Geometry check sheet. Reference: the model listing, model coordinates, mm. A direction names the side the tool comes from. Round coordinates to 2 decimals unless told otherwise and drop trailing zeros. Order: outer loops, then holes, each group sorted by start corner. A loop starts at its lowest first (then second) coordinate and runs counter-clockwise, first axis right, second up.
```python
from build123d import *

# Parameters (mm, degrees)
SKETCH_1_W          = 108
SKETCH_1_H          = 70
SKETCH_1_W_2        = 102
SKETCH_1_H_2        = 64
EXTRUDE_1_DEPTH     = 5
EXTRUDE_8_DEPTH     = 3
SKETCH_4_W          = 20
SKETCH_4_H          = 18
EXTRUDE_9_DEPTH     = 20
SKETCH_5_R          = 6.2
CUT_EXTRUDE_1_DEPTH = 76.7627877
FILLET_2_R          = 1
EXTRUDE_10_DEPTH    = 1
EXTRUDE_11_DEPTH    = 3
FILLET_3_R          = 3
SKETCH_8_R          = 10
CUT_EXTRUDE_2_DEPTH = 5
SKETCH_9_R          = 1
EXTRUDE_12_DEPTH    = 4
FILLET_4_R          = 3
FILLET_5_R          = 1
EXTRUDE_13_DEPTH    = 3
SKETCH_12_R         = 1
EXTRUDE_15_DEPTH    = 3


with BuildPart() as part:
    # 草图1 → 凸台-拉伸1 (new body)
    with BuildSketch(Plane(origin=(0, 0, 0), x_dir=(1, 0, 0), z_dir=(0, 1, 0))):
        Rectangle(SKETCH_1_W, SKETCH_1_H)
        Rectangle(SKETCH_1_W_2, SKETCH_1_H_2, mode=Mode.SUBTRACT)
    extrude(amount=EXTRUDE_1_DEPTH)

    # 草图3 → 凸台-拉伸8 (add)
    with BuildSketch(Plane.XZ):
        with BuildLine():
            Line((10, -35), (-10, -35))
            Line((-10, -35), (-10, -2))
            ThreePointArc((-10, -2), (-28.889417714, 19.435738798), (-54, 33.065106234))
            Line((-54, 33.065106234), (-54, 35))
            Line((-54, 35), (54, 35))
            Line((54, 35), (54, 33.065106234))
            ThreePointArc((54, 33.065106234), (28.889417714, 19.435738798), (10, -2))
            Line((10, -2), (10, -35))
        make_face()
    extrude(amount=EXTRUDE_8_DEPTH)

    # 草图4 → 凸台-拉伸9 (add)
    with BuildSketch(Plane(origin=(0, 0, -35), x_dir=(-1, 0, 0), z_dir=(0, 0, -1))):
        with Locations((0, -9)):
            Rectangle(SKETCH_4_W, SKETCH_4_H)
    extrude(amount=-EXTRUDE_9_DEPTH)

    # 草图5 → 切除-拉伸1 (cut, through all)
    with BuildSketch(Plane.XY.offset(-15)):
        with Locations((0, -10.5)):
            Circle(SKETCH_5_R)
    extrude(amount=-CUT_EXTRUDE_1_DEPTH, mode=Mode.SUBTRACT)

    # 圆角2
    # the kernel refuses this fillet: 1 mm, written as the material it adds along each edge
    with BuildSketch(Plane(origin=(-53.5, 0, 32), x_dir=(0, 1, 0), z_dir=(1, 0, 0))) as fillet_2_piece_1:
        with BuildLine():
            CenterArc((FILLET_2_R, -FILLET_2_R), FILLET_2_R, 90, 90)
            Line((0, -FILLET_2_R), (0, 0))
            Line((0, 0), (FILLET_2_R, 0))
        make_face()
    extrude(amount=107)

    # 草图6 → 凸台-拉伸10 (add)
    with BuildSketch(Plane(origin=(0, 0, 0), x_dir=(1, 0, 0), z_dir=(0, 1, 0))):
        Polygon((51, 32), (41, 32), (51, 22), align=None)
        Polygon((-51, 32), (-41, 32), (-51, 22), align=None)
        Polygon((-51, -22), (-51, -32), (-41, -32), align=None)
        Polygon((51, -32), (41, -32), (51, -22), align=None)
    extrude(amount=EXTRUDE_10_DEPTH)

    # 草图7 → 凸台-拉伸11 (add)
    with BuildSketch(Plane.XZ):
        Polygon((38, -35), (54, -19), (54, -35), align=None)
        Polygon((-54, -35), (-38, -35), (-54, -19), align=None)
        Polygon((54, 35), (38, 35), (54, 19), align=None)
        Polygon((-54, 35), (-38, 35), (-54, 19), align=None)
    extrude(amount=EXTRUDE_11_DEPTH)

    # 圆角3
    fillet_3_edges = [part.edges().sort_by_distance(p)[0] for p in [
        (44.013135699, -1.5, 28.986864301),
        (-44.013135699, -1.5, 28.986864301),
    ]]
    fillet(fillet_3_edges, radius=FILLET_3_R)

    # 草图8 → 切除-拉伸2 (cut, symmetric)
    with BuildSketch(Plane(origin=(0, 0, 0), x_dir=(1, 0, 0), z_dir=(0, 1, 0))):
        with Locations(Location((0, -20, 0), (0, 0, 270))):
            Circle(SKETCH_8_R)
    extrude(amount=CUT_EXTRUDE_2_DEPTH, both=True, mode=Mode.SUBTRACT)

    # 草图9 → 凸台-拉伸12 (add, symmetric)
    with BuildSketch(Plane(origin=(0, 1, 0), x_dir=(1, 0, 0), z_dir=(0, 1, 0))):
        with Locations(Location((46, -27, 0), (0, 0, 270))):
            Circle(SKETCH_9_R)
        with Locations(Location((-46, -27, 0), (0, 0, 315))):
            Circle(SKETCH_9_R)
        with Locations(Location((-46, 27, 0), (0, 0, 270))):
            Circle(SKETCH_9_R)
        with Locations(Location((46, 27, 0), (0, 0, 315))):
            Circle(SKETCH_9_R)
    extrude(amount=EXTRUDE_12_DEPTH, both=True)

    # 圆角4
    # the kernel refuses this fillet: 3 mm, written as the material it adds along each edge
    with BuildSketch(Plane(origin=(46.707106781, -3, 26.292893219), x_dir=(0.7071067811865442, 0, -0.7071067811865508), z_dir=(0, 1, 0)), Plane(origin=(-46.707106781, -3, -26.292893219), x_dir=(-0.7071067811865422, 0, 0.707106781186553), z_dir=(0, 1, 0))) as fillet_4_piece_1:
        with BuildLine():
            CenterArc((1.645751311, 3), FILLET_4_R, 228.590377891, 41.409622109)
            ThreePointArc((-0.338562172, 0.75), (-0.088562172, 0.411437828), (0, 0))
            Line((0, 0), (1.645751311, 0))
        make_face()
    extrude(amount=4)
    with BuildSketch(Plane(origin=(-46.707106781, -3, 26.292893219), x_dir=(0.9354143466934858, 0, -0.3535533905932727), z_dir=(0, 1, 0))) as fillet_4_piece_2:
        with BuildLine():
            CenterArc((2.057189139, 2.734313483), FILLET_4_R, 204.295188945, 41.409622109)
            Line((-0.677124344, 1.5), (0, 0))
            ThreePointArc((0, 0), (0.411437828, 0.088562172), (0.822875656, 0))
        make_face()
    extrude(amount=4)
    with BuildSketch(Plane(origin=(-45.292893219, -3, -27.707106781), x_dir=(0.7071067811865529, 0, -0.7071067811865421), z_dir=(0, 1, 0)), Plane(origin=(46.707106781, -3, -26.292893219), x_dir=(0.7071067811865476, 0, 0.7071067811865476), z_dir=(0, 1, 0))) as fillet_4_piece_3:
        with BuildLine():
            CenterArc((1.645751311, -3), FILLET_4_R, 90, 41.409622109)
            ThreePointArc((-0.338562172, -0.75), (-0.088562172, -0.411437828), (0, 0))
            Line((0, 0), (1.645751311, 0))
        make_face()
    extrude(amount=4)
    with BuildSketch(Plane(origin=(45.292893219, -3, -27.707106781), x_dir=(-0.35355339059328167, 0, 0.9354143466934823), z_dir=(0, 1, 0))) as fillet_4_piece_4:
        with BuildLine():
            CenterArc((2.057189139, -2.734313483), FILLET_4_R, 114.295188945, 41.409622109)
            Line((-0.677124344, -1.5), (0, 0))
            ThreePointArc((0, 0), (0.411437828, -0.088562172), (0.822875656, 0))
        make_face()
    extrude(amount=4)

    # 圆角5
    fillet_5_edges = [part.edges().sort_by_distance(p)[0] for p in [
        (46, 5, 26),
        (-46.707106781, 5, 26.292893219),
        (-46, 5, -28),
        (45.292893219, 5, -27.707106781),
    ]]
    fillet(fillet_5_edges, radius=FILLET_5_R)

    # 草图10 → 凸台-拉伸13 (add)
    with BuildSketch(Plane.XZ):
        Polygon((-51, 22), (-54, 19), (-54, -19), (-51, -22), align=None)
        Polygon((54, -19), (51, -22), (51, 22), (54, 19), align=None)
    extrude(amount=EXTRUDE_13_DEPTH)

    # 草图12 → 凸台-拉伸15 (add)
    with BuildSketch(Plane.XZ.offset(3)):
        with Locations(Location((0, -8, 0), (0, 0, 90))):
            Circle(SKETCH_12_R)
        with Locations(Location((0, 8, 0), (0, 0, 90))):
            Circle(SKETCH_12_R)
    extrude(amount=EXTRUDE_15_DEPTH)


solid = part.part
```
(1) Draft check along X on faces 6 (the cylindrical face through (1, -4, 8)), 7 (the flat face through (-4, 5, 34)), 8 (the cylindrical face through (43.726, -1.479, 28.316)). Enter one of: released by +X, released by -X, zero draft, split by the parting line, or undercut.
Returned:
face 6: split by the parting line
face 7: zero draft
face 8: undercut
(2) Depth check by flat-ended pin: P1, Ø2.5, axis at x = 32.5, z = -33, coming from the -Y side; P2, Ø5.5, axis at y = -10, z = -19, coming from the +X side; P3, Ø12, axis at x = -4, z = 25.5, coming from the +Y side. Enter the tip coordinate at first touch or a pass-through.
Returned:
P1: stops at y = 0
P2: stops at x = 10
P3: stops at y = 0.13
(3) Sectioned sample at C-C, the plane z = 20. Record the cut outline in (x, y).
Returned:
outline: (-54, -3) - (-51, -3) - (-51, 5) - (-54, 5) - close; (-29.61, -3) - (-10, -3) - (-10, 0) - (-29.61, 0) - close; (10, -3) - (29.61, -3) - (29.61, 0) - (10, 0) - close; (51, -3) - (54, -3) - (54, 5) - (51, 5) - close
(4) Set-up check for faces 1 (the flat face through (49, -1, -24)), 2 (the flat face through (-10, -9, -22)), 3 (the flat face through (-41, -1, -32)), 4 (the flat face through (0, -6, -8)), 5 (the flat face through (-1, 2, -32)): record each of +Z, -Z, +X, -X, +Y, -Y from which the full face is reachable in a straight line by a thin tool's end or side.
Returned:
face 1: +Y, -Y
face 2: -Z, -Y
face 3: -Y
face 4: +Z, -Z, +X, -X, -Y
face 5: +Y
(5) Sectioned sample at A-A, the plane x = 29. Record the cut outline in (y, z), and give its area (3 significant figures).
Returned:
outline: (-3, 19.52) - (0, 19.52) - (0, 31) arc R1 cw to (1, 32) - (5, 32) - (5, 35) - (-3, 35) - close; (0, -35) - (5, -35) - (5, -32) - (0, -32) - close
area: 76.6 mm2
(6) Material ranges on line 1 (X direction, y = -1.5, z = -22.5); line 2 (Y direction, x = 0, z = -20.5); line 3 (Z direction, x = 14, y = 4), recorded low to high.
Returned:
line 1: x = -54 to -50.5, -10 to 10, 50.5 to 54
line 2: y = -18 to -16.7, -4.3 to 0
line 3: z = -35 to -32, 32 to 35
(7) Sectioned sample at D-D, the plane y = -15.5. Record the cut outline in (x, z).
Returned:
outline: (-10, -35) - (-3.67, -35) - (-3.67, -15) - (-10, -15) - close; (3.67, -35) - (10, -35) - (10, -15) - (3.67, -15) - close
